Source: CAD feature listing. Evaluate the final solid. Frame: model axes, mm. A direction names the side the tool comes from. Round coordinates to 2 decimals unless told otherwise and drop trailing zeros. Order: outer loops, then holes, each group sorted by start corner. A loop starts at its lowest first (then second) coordinate and runs counter-clockwise, first axis right, second up. Notation, with made-up numbers: (83, 1.25) - (109, 1.25) arc R29 ccw to (109, 38.25) - close; hole circle Ø1 at (35, 63). An arc over 180 degrees is marked (long way). Return JSON: item names as keys, results as strings. Group by question number.
1) Section D-D, the plane z = -7.25. Return loops of the section in (x, y).
2) Ray query, line 1 (X direction, y = 7, z = -5); line 2 (Z direction, x = 0.5, y = 7.25); line 3 (Z direction, x = -8.5, y = 1.75). Return the intervals inside material, ascending. Write a range as from..to.
3) Section B-B, the plane z = -2.5. Return loops of the section in (x, y).
4) Section C-C, the plane x = 4.75. Return loops of the section in (y, z), plus the area to 3 significant figures.
5) Contact query for flat-ended pins moving along their axis: P1, Ø2.5, axis at y = 5.5, z = 4.5, coming from the +X side; P2, Ø1, axis at y = 2.5, z = 7.5, coming from the -X side; P3, Ø3, axis at x = 13.95, y = 4, coming from the +Z side; P4, Ø1.8, axis at x = -10.05, y = 4, coming from the -Z side. Output: stop coordinate, or through.
6) Access query for faces 1 (the flat face through (9, 7, -5.801)), 2 (the flat face through (11, 4, -4.301)), 3 (the cylindrical face through (5.14, 2.45, -9.79)). Directions: +Z, -Z, +X, -X, +Y, -Y. A direction counts if a zero-diameter tool reaches every point of the face in a straight line with its end or side. Return the directions, or none.
7) Section A-A, the plane x = -0.5. Return loops of the section in (y, z).
```python
from build123d import *

# Parameters (mm, degrees)
SKETCH1_W           = 4
SKETCH1_H           = 1
BOSS_EXTRUDE3_DEPTH = 8
SKETCH2_R           = 4
BOSS_EXTRUDE5_DEPTH = 3
SKETCH3_R           = 2.5
BOSS_EXTRUDE6_DEPTH = 3
SKETCH4_R           = 1
CUT_EXTRUDE1_DEPTH  = 23.259998772
FILLET2_R           = 1
FILLET3_R           = 1
SKETCH6_R           = 1.75
BOSS_EXTRUDE8_DEPTH = 2


with BuildPart() as part:
    # Sketch1 → Boss-Extrude3 (new body)
    with BuildSketch(Plane(origin=(0, 0, 0), x_dir=(1, 0, 0), z_dir=(0, 1, 0))):
        Polygon((9.951219512, 4.301393728), (9.951219512, 5.801393728), (-8.048780488, 5.801393728), (-8.048780488, -11.198606272), (11.951219512, -11.198606272), (11.951219512, 4.301393728), align=None)
        with Locations((13.951219512, 1.608013937)):
            Rectangle(SKETCH1_W, SKETCH1_H)
        with Locations((-10.048780488, 1.608013937)):
            Rectangle(SKETCH1_W, SKETCH1_H)
    extrude(amount=BOSS_EXTRUDE3_DEPTH)

    # Sketch2 → Boss-Extrude5 (add)
    with BuildSketch(Plane(origin=(0, 0, -5.801393728), x_dir=(-1, 0, 0), z_dir=(0, 0, -1))):
        with Locations(Location((-5.951219512, 4, 0), (0, 0, 180))):
            Circle(SKETCH2_R)
    extrude(amount=BOSS_EXTRUDE5_DEPTH)

    # Sketch3 → Boss-Extrude6 (add)
    with BuildSketch(Plane(origin=(0, 0, -5.801393728), x_dir=(-1, 0, 0), z_dir=(0, 0, -1))):
        with Locations((-0.951219512, 3.925831124)):
            Circle(SKETCH3_R)
    extrude(amount=BOSS_EXTRUDE6_DEPTH)

    # Sketch4 → Cut-Extrude1 (cut, through all)
    with BuildSketch(Plane(origin=(0, 0, -2.108013937), x_dir=(-1, 0, 0), z_dir=(0, 0, -1))):
        with Locations((-13.951219512, 4)):
            Circle(SKETCH4_R)
        with Locations((10.048780488, 4)):
            Circle(SKETCH4_R)
    extrude(amount=-CUT_EXTRUDE1_DEPTH, mode=Mode.SUBTRACT)

    # Fillet2
    fillet2_edges = [part.edges().sort_by_distance(p)[0] for p in [
        (15.951219512, 8, -1.608013937),
    ]]
    fillet(fillet2_edges, radius=FILLET2_R)

    # Fillet3
    fillet3_edges = [part.edges().sort_by_distance(p)[0] for p in [
        (15.951219512, 0, -1.608013937),
        (-12.048780488, 8, -1.608013937),
        (-12.048780488, 0, -1.608013937),
    ]]
    fillet(fillet3_edges, radius=FILLET3_R)

    # Sketch6 → Boss-Extrude8 (add)
    with BuildSketch(Plane(origin=(0, 0, -8.801393728), x_dir=(-1, 0, 0), z_dir=(0, 0, -1))):
        with Locations((-5.951219512, 4)):
            Circle(SKETCH6_R)
    extrude(amount=BOSS_EXTRUDE8_DEPTH)


solid = part.part
```
Geometry check:
{
 "1": {"outline": "(2.45, 5.93) arc R2.5 ccw (long way) to (2.51, 1.97) arc R4 ccw (long way) to start"},
 "2": {"line 1": "-8.05..9.95", "line 2": "-5.8..11.2", "line 3": "-2.11..-1.11"},
 "3": {"outline": "(-8.05, 0) - (11.95, 0) - (11.95, 8) - (-8.05, 8) - close"},
 "4": {"outline": "(0, -5.8) - (0.18, -5.8) - (0.18, -8.8) - (2.73, -8.8) - (2.73, -10.8) - (5.27, -10.8) - (5.27, -8.8) - (7.82, -8.8) - (7.82, -5.8) - (8, -5.8) - (8, 11.2) - (0, 11.2) - close", "area": "164 mm2"},
 "5": {"P1": "x = 11.95", "P2": "x = -8.05", "P3": "z = -1.11", "P4": "through"},
 "6": {"face 1": "-Z, +X, +Y", "face 2": "-Z, +X, +Y, -Y", "face 3": "-Z"},
 "7": {"outline": "(0, -5.8) - (1.89, -5.8) - (1.89, -8.8) - (5.96, -8.8) - (5.96, -5.8) - (8, -5.8) - (8, 11.2) - (0, 11.2) - close"}
}
